from build123d import *

# Parameters (mm, degrees)
BOSS_EXTRUDE1_DEPTH     = 5
SKETCH3_R               = 1.5
CUT_EXTRUDE1_DEPTH      = 10
CUT_EXTRUDE2_REACH      = 7
CUT_EXTRUDE4_DEPTH      = 10
CUT_EXTRUDE5_DEPTH      = 10
CUT_EXTRUDE5_DEPTH_BACK = 10
CUT_EXTRUDE6_DEPTH      = 10
SKETCH8_W               = 3.5
SKETCH8_H               = 3
CUT_EXTRUDE13_DEPTH     = 1.1
SKETCH9_W               = 3.5
SKETCH9_H               = 3
CUT_EXTRUDE14_DEPTH     = 1.1


with BuildPart() as part:
    # Sketch1 → Boss-Extrude1 (new body)
    with BuildSketch(Plane(origin=(0, 0, 0), x_dir=(1, 0, 0), z_dir=(0, 1, 0))):
        Polygon((-5, 5), (-5, -5), (5, -5), (5, 5), (2.5, 5), (1e-09, 5), (-2.5, 5), align=None)
        with BuildLine():
            Line((-2.5, 7.5), (-2.5, 5))
            Line((-2.5, 5), (1e-09, 5))
            ThreePointArc((1e-09, 5), (-1.767766953, 5.732233047), (-2.5, 7.5))
        make_face()
        with BuildLine():
            Line((1e-09, 5), (2.5, 5))
            Line((2.5, 5), (2.5, 7.5))
            ThreePointArc((2.5, 7.5), (1.767766953, 5.732233047), (1e-09, 5))
        make_face()
        with BuildLine():
            ThreePointArc((2.5, 7.5), (0, 10), (-2.5, 7.5))
            Line((-2.5, 7.5), (-1.5, 7.5))
            Line((-1.5, 7.499999998), (-1.5, 8))
            Line((-1.5, 8), (-1.414213562, 8))
            ThreePointArc((-1.414213562, 8), (-1.060660172, 8.560660172), (-0.5, 8.914213562))
            Line((-0.5, 8.914213562), (-0.5, 9))
            Line((-0.5, 9), (-1.7e-08, 9))
            Line((-1.7e-08, 9), (0.5, 9))
            Line((0.5, 9), (0.5, 8.914213562))
            ThreePointArc((0.5, 8.914213562), (1.060660172, 8.560660172), (1.414213562, 8))
            Line((1.414213562, 8), (1.5, 8))
            Line((1.5, 8), (1.5, 7.5))
            Line((1.5, 7.5), (2.5, 7.5))
        make_face()
        with BuildLine():
            ThreePointArc((-2.5, 7.5), (-1.767766953, 5.732233047), (1e-09, 5))
            ThreePointArc((1e-09, 5), (1.767766953, 5.732233047), (2.5, 7.5))
            Line((2.5, 7.5), (1.5, 7.5))
            Line((1.5, 7.5), (1.5, 7))
            Line((1.5, 7), (1.414213562, 7))
            ThreePointArc((1.414213562, 7), (1.060660172, 6.439339828), (0.5, 6.085786438))
            Line((0.5, 6.085786438), (0.5, 6))
            Line((0.5, 6), (0, 6))
            Line((0, 6), (-0.5, 6))
            Line((-0.5, 6), (-0.5, 6.085786438))
            ThreePointArc((-0.5, 6.085786438), (-1.060660172, 6.439339828), (-1.414213562, 7))
            Line((-1.414213562, 7), (-1.5, 7))
            Line((-1.5, 7), (-1.5, 7.499999998))
            Line((-1.5, 7.5), (-2.5, 7.5))
        make_face()
        with BuildLine():
            Line((0.5, 6), (0.5, 6.085786438))
            ThreePointArc((0.5, 6.085786438), (0.253652968, 6.021602161), (0, 6))
            Line((0, 6), (0.5, 6))
        make_face()
        with BuildLine():
            Line((-0.5, 7), (-1.414213562, 7))
            ThreePointArc((-1.414213562, 7), (-1.060660172, 6.439339828), (-0.5, 6.085786438))
            Line((-0.5, 6.085786438), (-0.5, 7))
        make_face()
        with BuildLine():
            ThreePointArc((0.5, 6.085786438), (1.060660172, 6.439339828), (1.414213562, 7))
            Line((1.414213562, 7), (0.5, 7))
            Line((0.5, 7), (0.5, 6.085786438))
        make_face()
        with BuildLine():
            Line((0.5, 8), (1.414213562, 8))
            ThreePointArc((1.414213562, 8), (1.060660172, 8.560660172), (0.5, 8.914213562))
            Line((0.5, 8.914213562), (0.5, 8))
        make_face()
        with BuildLine():
            ThreePointArc((-0.5, 8.914213562), (-1.060660172, 8.560660172), (-1.414213562, 8))
            Line((-1.414213562, 8), (-0.5, 8))
            Line((-0.5, 8), (-0.5, 8.914213562))
        make_face()
        with BuildLine():
            Line((-0.5, 9), (-0.5, 8.914213562))
            ThreePointArc((-0.5, 8.914213562), (-0.253652976, 8.978397838), (-1.7e-08, 9))
            Line((-1.7e-08, 9), (-0.5, 9))
        make_face()
        with BuildLine():
            ThreePointArc((-1.7e-08, 9), (0.25365296, 8.978397841), (0.5, 8.914213562))
            Line((0.5, 8.914213562), (0.5, 9))
            Line((0.5, 9), (-1.7e-08, 9))
        make_face()
        with BuildLine():
            ThreePointArc((-1.414213562, 7), (-1.478397839, 7.246347031), (-1.5, 7.499999998))
            Line((-1.5, 7.499999998), (-1.5, 7))
            Line((-1.5, 7), (-1.414213562, 7))
        make_face()
        with BuildLine():
            ThreePointArc((0, 6), (-0.253652968, 6.021602161), (-0.5, 6.085786438))
            Line((-0.5, 6.085786438), (-0.5, 6))
            Line((-0.5, 6), (0, 6))
        make_face()
        with BuildLine():
            Line((-1.5, 8), (-1.5, 7.499999998))
            ThreePointArc((-1.5, 7.499999998), (-1.47839784, 7.753652967), (-1.414213562, 8))
            Line((-1.414213562, 8), (-1.5, 8))
        make_face()
        with BuildLine():
            Line((1.5, 7), (1.5, 7.5))
            ThreePointArc((1.5, 7.5), (1.478397839, 7.246347032), (1.414213562, 7))
            Line((1.414213562, 7), (1.5, 7))
        make_face()
        with BuildLine():
            ThreePointArc((1.414213562, 8), (1.478397839, 7.753652968), (1.5, 7.5))
            Line((1.5, 7.5), (1.5, 8))
            Line((1.5, 8), (1.414213562, 8))
        make_face()
    extrude(amount=BOSS_EXTRUDE1_DEPTH)

    # Sketch2 → Cut-Revolve3 (revolve, cut)
    with BuildSketch(Plane(origin=(0, 0, 0), x_dir=(0, 0, -1), z_dir=(1, 0, 0))):
        with BuildLine():
            Line((-2.5, 5.5), (-2.5, -0.5))
            ThreePointArc((-2.5, -0.5), (0.5, 2.5), (-2.5, 5.5))
        make_face()
    revolve(axis=Axis((0, 5.5, 2.5), (0, -1, 0)), mode=Mode.SUBTRACT)

    # Sketch3 → Cut-Extrude1 (cut)
    with BuildSketch(Plane(origin=(5, 0, 0), x_dir=(0, 0, -1), z_dir=(1, 0, 0))):
        with Locations((-2.5, 2.5)):
            Circle(SKETCH3_R)
    extrude(amount=-CUT_EXTRUDE1_DEPTH, mode=Mode.SUBTRACT)

    # Sketch4 → Cut-Extrude2 (cut, up to next)
    with BuildSketch(Plane(origin=(0, 5, 0), x_dir=(1, 0, 0), z_dir=(0, 1, 0)), mode=Mode.PRIVATE) as cut_extrude2_sk1:
        Polygon((-5, 0), (-3.5, -5), (-5, -5), align=None)
    cut_extrude2_tool1 = extrude(cut_extrude2_sk1.sketch, amount=-CUT_EXTRUDE2_REACH, mode=Mode.PRIVATE) & part.part
    add(cut_extrude2_tool1.solids().sort_by_distance((-4.5, 5, 3.333333))[0], mode=Mode.SUBTRACT)
    # Sketch4 → Cut-Extrude2 (cut, up to next)
    with BuildSketch(Plane(origin=(0, 5, 0), x_dir=(1, 0, 0), z_dir=(0, 1, 0)), mode=Mode.PRIVATE) as cut_extrude2_sk2:
        Polygon((5, 0), (3.5, -5), (5, -5), align=None)
    cut_extrude2_tool2 = extrude(cut_extrude2_sk2.sketch, amount=-CUT_EXTRUDE2_REACH, mode=Mode.PRIVATE) & part.part
    add(cut_extrude2_tool2.solids().sort_by_distance((4.5, 5, 3.333333))[0], mode=Mode.SUBTRACT)

    # Sketch5 → Cut-Extrude4 (cut)
    with BuildSketch(Plane(origin=(0, 5, 0), x_dir=(1, 0, 0), z_dir=(0, 1, 0))):
        with BuildLine():
            ThreePointArc((-1.658312395, -2.5), (0, -0.841687605), (1.658312395, -2.5))
            Line((1.658312395, -2.5), (2.5, -2.5))
            ThreePointArc((2.5, -2.5), (0, 0), (-2.5, -2.5))
            Line((-2.5, -2.5), (-1.658312395, -2.5))
        make_face()
        with BuildLine():
            Line((2.5, -2.5), (1.658312395, -2.5))
            ThreePointArc((1.658312395, -2.5), (0, -4.158312395), (-1.658312395, -2.5))
            Line((-1.658312395, -2.5), (-2.5, -2.5))
            ThreePointArc((-2.5, -2.5), (-1.767766953, -4.267766953), (0, -5))
            ThreePointArc((0, -5), (1.767766953, -4.267766953), (2.5, -2.5))
        make_face()
        with BuildLine():
            Line((2.5, -5), (2.5, -2.5))
            ThreePointArc((2.5, -2.5), (1.767766953, -4.267766953), (0, -5))
            Line((0, -5), (2.5, -5))
        make_face()
        with BuildLine():
            ThreePointArc((0, -5), (-1.767766953, -4.267766953), (-2.5, -2.5))
            Line((-2.5, -2.5), (-2.5, -5))
            Line((-2.5, -5), (0, -5))
        make_face()
    extrude(amount=-CUT_EXTRUDE4_DEPTH, mode=Mode.SUBTRACT)

    # Sketch6 → Cut-Extrude5 (cut, two sides)
    with BuildSketch(Plane(origin=(-2.5, 0, 0), x_dir=(0, 0, -1), z_dir=(1, 0, 0))) as cut_extrude5_sk:
        with BuildLine():
            ThreePointArc((-5, 2.5), (-4.267766953, 4.267766953), (-2.5, 5))
            Line((-2.5, 5), (-5, 5))
            Line((-5, 5), (-5, 2.5))
        make_face()
        with BuildLine():
            Line((-5, 0), (-2.5, 0))
            ThreePointArc((-2.5, 0), (-4.267766953, 0.732233047), (-5, 2.5))
            Line((-5, 2.5), (-5, 0))
        make_face()
    extrude(amount=CUT_EXTRUDE5_DEPTH, mode=Mode.SUBTRACT)
    extrude(cut_extrude5_sk.sketch, amount=-CUT_EXTRUDE5_DEPTH_BACK, mode=Mode.SUBTRACT)

    # Sketch7 → Cut-Extrude6 (cut)
    with BuildSketch(Plane.ZY.offset(5)):
        with BuildLine():
            Line((-3.914213562, 2), (-3, 2))
            Line((-3, 2), (-3, 3))
            Line((-3, 3), (-3.914213562, 3))
            ThreePointArc((-3.914213562, 3), (-3.978397839, 2.753652968), (-4, 2.5))
            ThreePointArc((-4, 2.5), (-3.978397839, 2.246347032), (-3.914213562, 2))
        make_face()
        Polygon((-3, 3), (-3, 2), (-2, 3), align=None)
        with BuildLine():
            Line((-3, 3), (-2, 3))
            Line((-2, 3), (-2, 3.914213562))
            ThreePointArc((-2, 3.914213562), (-2.246347032, 3.978397839), (-2.5, 4))
            ThreePointArc((-2.5, 4), (-2.753652968, 3.978397839), (-3, 3.914213562))
            Line((-3, 3.914213562), (-3, 3))
        make_face()
        Polygon((-2, 3), (-3, 2), (-2, 2), align=None)
        with BuildLine():
            Line((-1.085786438, 3), (-2, 3))
            Line((-2, 3), (-2, 2))
            Line((-2, 2), (-1.085786438, 2))
            ThreePointArc((-1.085786438, 2), (-1.021602161, 2.246347032), (-1, 2.5))
            ThreePointArc((-1, 2.5), (-1.021602161, 2.753652968), (-1.085786438, 3))
        make_face()
        with BuildLine():
            Line((-2, 2), (-3, 2))
            Line((-3, 2), (-3, 1.085786438))
            ThreePointArc((-3, 1.085786438), (-2.753652968, 1.021602161), (-2.5, 1))
            ThreePointArc((-2.5, 1), (-2.246347032, 1.021602161), (-2, 1.085786438))
            Line((-2, 1.085786438), (-2, 2))
        make_face()
    extrude(amount=-CUT_EXTRUDE6_DEPTH, mode=Mode.SUBTRACT)

    # Sketch8 → Cut-Extrude13 (cut)
    with BuildSketch(Plane(origin=(0, 5, 0), x_dir=(1, 0, 0), z_dir=(0, 1, 0))):
        with Locations((2.25, 2.5)):
            Rectangle(SKETCH8_W, SKETCH8_H)
        with Locations((-2.25, 2.5)):
            Rectangle(SKETCH8_W, SKETCH8_H)
    extrude(amount=-CUT_EXTRUDE13_DEPTH, mode=Mode.SUBTRACT)

    # Sketch9 → Cut-Extrude14 (cut)
    with BuildSketch(Plane(origin=(0, 0, 0), x_dir=(-1, 0, 0), z_dir=(0, -1, 0))):
        with Locations((-2.25, 2.5)):
            Rectangle(SKETCH9_W, SKETCH9_H)
        with Locations((2.25, 2.5)):
            Rectangle(SKETCH9_W, SKETCH9_H)
    extrude(amount=-CUT_EXTRUDE14_DEPTH, mode=Mode.SUBTRACT)


solid = part.part
Source: CAD feature listing. Evaluate the final solid. Frame: model axes, mm. A direction names the side the tool comes from. Give positions to 0.01 mm unless a question says otherwise; leave off trailing zeros. Write each loop counter-clockwise with the first axis right and the second up, starting at its lowest first coordinate (ties: lowest second). Pieces come first, ordered by that corner, then holes. Notation, with made-up numbers: (11.5, -24) -> (20.5, -24) arc R19 ccw to (20.5, -5) -> close; hole circle Ø10 at (11, 27). An arc over 180 degrees is marked (long way). Return JSON: item names as keys, results as strings. Group by question number.
1. Material intervals for line 1 (X direction, y = 4.4, z = -3.5); line 2 (Z direction, x = 4.5, y = 2.6); line 3 (Z direction, x = 3, y = 2.5), sorted ascending. Write a range as from..to.
2. Section A-A, the plane x = -3. Output: boundary loops of the cut face in (y, z).
3. Section B-B, the plane z = 1.5. Output: boundary loops of the cut face in (x, y), then the cut area to 3 significant figures.
4. Access query for faces 5 (the face through (-0.1, 1.5, -3)), 6 (the face through (-1, 2, -7)), 7 (the face through (-2.5, 3.1, 4.3)), 8 (the face through (4, 0.5, -2.5)), 9 (the face through (2.2, 4.5, -1)). Directions: +Z, -Z, +X, -X, +Y, -Y. A direction counts if a zero-diameter tool reaches every point of the face in a straight line with its end or side. Return the directions, or none.
5. Pin query (flat end, axial travel): pin 1 Ø3 at (y, z) = (3.5, 3) entering from -X; pin 2 Ø0.7 at (x, y) = (-1, 2) entering from +Z; pin 3 Ø1 at (y, z) = (2.5, -7) entering from -X. Return the tip coordinate at first contact, or that it passes through.
6. Mould query, pull axis Z, two halves, no side actions, for faces 1 (the face through (0.1, 0.4, 0)), 2 (the face through (2.5, 2.54, 4.32)), 3 (the face through (4, 2, -5)), 4 (the face through (-0.1, 2, -1.5)). Classes: +Z half, -Z half, draft (parallel to the pull), parting line (faces both ways), or undercut.
7. Section C-C, the plane z = -8.5. Output: boundary loops of the cut face in (x, y).
8. Section D-D, the plane x = -1.25. Count the separate pieces of the cut face and the enclosed holes in it, then the cut area to 3 significant figures.
Determined:
{
 "1": {"line 1": "x = -5..-4, -0.5..0.5, 4..5", "line 2": "z = -5..-4, -1..1", "line 3": "z = -5..-4, -1..1, 4..5"},
 "2": {"outline": "(0, -5) -> (5, -5) -> (5, -4) -> (3.9, -4) -> (3.9, -3) -> (3, -3) -> (3, -3.91) arc R1.5 cw to (2, -3.91) -> (2, -3) -> (1.1, -3) -> (1.1, -4) -> (0, -4) -> close; (0, -1) -> (1.1, -1) -> (1.1, -2) -> (2, -2) -> (2, -1.09) arc R1.5 cw to (3, -1.09) -> (3, -2) -> (3.9, -2) -> (3.9, -1) -> (5, -1) -> (5, 2.5) arc R2.5 ccw to (0, 2.5) -> close; hole circle Ø3 at (2.5, 2.5)"},
 "3": {"outline": "(-4.55, 0) -> (-2.29, 0) -> (-2.29, 0.84) arc R2.83 cw to (-2.6, 1.38) -> (-4.55, 1.38) -> close; (-4.55, 3.62) -> (-2.6, 3.62) arc R2.83 cw to (-2.29, 4.16) -> (-2.29, 5) -> (-4.55, 5) -> close; (2.29, 0) -> (4.55, 0) -> (4.55, 1.38) -> (2.6, 1.38) arc R2.83 cw to (2.29, 0.84) -> close; (2.29, 4.16) arc R2.83 cw to (2.6, 3.62) -> (4.55, 3.62) -> (4.55, 5) -> (2.29, 5) -> close", "area": "12.1 mm2"},
 "4": {"face 5": "+X, -X", "face 6": "+Y, -Y", "face 7": "+Z, +Y, -Y", "face 8": "-Y", "face 9": "+Y"},
 "5": {"pin 1": "stops at x = -4.55", "pin 2": "stops at z = -0.12", "pin 3": "stops at x = -2.5"},
 "6": {"face 1": "+Z half", "face 2": "draft", "face 3": "-Z half", "face 4": "undercut"},
 "7": {"outline": "(-2.29, 0) -> (-0.5, 0) -> (-0.5, 5) -> (-2.29, 5) -> close; (0.5, 0) -> (2.29, 0) -> (2.29, 5) -> (0.5, 5) -> close"},
 "8": {"separate pieces": "3", "enclosed holes": "0", "area": "32.4 mm2"}
}
